Autodesk Inventor part; units mm, degrees
ref_plane "YZ Plane" through (0, 0, 0) normal (1, 0, 0) x (0, 1, 0)
ref_plane "XZ Plane" through (0, 0, 0) normal (0, 1, 0) x (-1, 0, 0)
ref_plane "XY Plane" through (0, 0, 0) normal (0, 0, 1) x (1, 0, 0)
sketch "Sketch1" plane through (0, 0, 0) normal (0, 0, 1) x (1, 0, 0)
  line L0 (0, 0) -> (-5, 0)
  line L1 (-5, 0) -> (-5, -5)
  line L2 (-5, -5) -> (0, -5)
  line L3 (0, -5) -> (0, 0)
  line L4 (-40, 0) -> (-35, 0)
  line L5 (-35, 0) -> (-35, -5)
  line L6 (-35, -5) -> (-40, -5)
  line L7 (-40, -5) -> (-40, 0)
  line L8 (0, -15.1) -> (-5, -15.1)
  line L9 (-5, -15.1) -> (-5, -10.1)
  line L10 (-5, -10.1) -> (0, -10.1)
  line L11 (0, -10.1) -> (0, -15.1)
  line L12 (-40, -15.1) -> (-35, -15.1)
  line L13 (-35, -15.1) -> (-35, -10.1)
  line L14 (-35, -10.1) -> (-40, -10.1)
  line L15 (-40, -10.1) -> (-40, -15.1)
  line L16 (0, 0) -> (-5, 0)
  line L17 (-35, 0) -> (-40, 0)
  line L18 (0, -15.1) -> (0, -10.1)
  line L19 (0, -5) -> (0, 0)
  line L20 (-40, -15.1) -> (-35, -15.1)
  line L21 (-5, -15.1) -> (0, -15.1)
  line L22 (-40, 0) -> (-40, -5)
  line L23 (-40, -10.1) -> (-40, -15.1)
  dimension "d0" = 40
  dimension "d1" = 15.1
  dimension "d2" = 5
  dimension "d3" = 5
  dimension "d4" = 5
  dimension "d5" = 5
  dimension "d6" = 5
  dimension "d7" = 5
  dimension "d8" = 5
  dimension "d9" = 5
extrude "Mounting arms" add sketch "Sketch1" along normal blind 15
sketch "Sketch2" plane through (0, 0, 0) normal (0, 0, -1) x (-1, 0, 0)
  line L0 (-19.9999, -1.0001) -> (59.9998, -1.0001)
  line L1 (59.9998, -1.0001) -> (59.9998, -14.0997)
  line L2 (59.9998, -14.0997) -> (-19.9999, -14.0997)
  line L3 (-19.9999, -14.0997) -> (-19.9999, -1.0001)
  point P0 (0, 0)
extrude "Plate" add sketch "Sketch2" along normal blind 2.5
sketch "Sketch3" plane through (19.9999, -14.0997, 0) normal (1, 0, 0) x (0, 0, -1)
  circle A0 centre (6, 6.5498) radius 5
  point P0 (0, 14.0997)
  dimension "d14" = 10
sketch "Sketch5" plane through (-59.9998, -14.0997, 0) normal (-1, 0, 0) x (0, 0, 1)
  circle A0 centre (-6, 6.5498) radius 5
  point P0 (0, 14.0997)
  dimension "d15" = 10
extrude "retainer1" add sketch "Sketch5" against normal blind 4
extrude "retainer2" add sketch "Sketch3" against normal blind 4
sketch "Sketch6" plane through (-59.9998, -14.0997, 0) normal (-1, 0, 0) x (0, 0, 1)
  line L0 (0, 13.0996) -> (0, 0)
  circle A0 centre (-5.9997, 6.4943) radius 3.5
  point P0 (0, 14.0997)
  dimension "d21" = 7
extrude "cyldiner shaft holes" cut sketch "Sketch6" against normal blind 80
chamfer "Chamfer1" distance 1 angle 45 2 edges at (-37.5, 0, 0) (-2.5, 0, 0)
sketch "Sketch7" plane through (0, 0, 15) normal (0, 0, 1) x (1, 0, 0)
  line L0 (-40, -1.0001) -> (-40, -5)
  line L1 (0, -14.0997) -> (0, -10.1)
  line L2 (-35, -14.0997) -> (-35, -10.1)
  line L3 (-40, -12.6005) -> (-35, -12.6005)
  line L4 (-35, -12.6005) -> (-35, -10.1)
  line L5 (-35, -10.1) -> (-40, -10.1)
  line L6 (-40, -10.1) -> (-40, -12.6005)
  line L7 (-5, -10.1) -> (-5, -15.1)
  line L8 (0, -12.6005) -> (-5, -12.6005)
  line L9 (-5, -12.6005) -> (-5, -10.1)
  line L10 (-5, -10.1) -> (0, -10.1)
  line L11 (0, -10.1) -> (0, -12.6005)
  line L12 (-5, -5) -> (0, -5)
  line L13 (0, -2.5001) -> (-5, -2.5001)
  line L14 (-5, -2.5001) -> (-5, -5)
  line L15 (-5, -5) -> (0, -5)
  line L16 (0, -5) -> (0, -2.5001)
  line L17 (-40, -2.5001) -> (-35, -2.5001)
  line L18 (-35, -2.5001) -> (-35, -5)
  line L19 (-35, -5) -> (-40, -5)
  line L20 (-40, -5) -> (-40, -2.5001)
  line L21 (-40, -2.5001) -> (-35, -2.5001)
  line L22 (-5, -2.5001) -> (0, -2.5001)
  line L23 (-40, -12.6005) -> (-40, -10.1)
  line L24 (-40, -5) -> (-40, -2.5001)
  line L25 (0, -12.6005) -> (-5, -12.6005)
  line L26 (-35, -12.6005) -> (-40, -12.6005)
  line L27 (0, -2.5001) -> (0, -5)
  line L28 (0, -10.1) -> (0, -12.6005)
  point P0 (0, 0)
extrude "Extrusion6" add sketch "Sketch7" along normal blind 5
fillet "Fillet1" radius 1 24 edges at (-35, -2.5001, 17.5) (-40, -2.5001, 17.5) (-37.5, -2.5001, 20) (-5, -2.5001, 17.5) (0, -2.5001, 17.5) (-2.5, -2.5001, 20) (0, -12.6005, 17.5) (-2.5, -12.6005, 20) (-5, -12.6005, 17.5) (-35, -12.6005, 17.5) (-37.5, -12.6005, 20) (-40, -12.6005, 17.5) (0, 0, 8) (-5, 0, 8) (-2.5, 0, 15) (-35, 0, 8) (-37.5, 0, 15) (-40, 0, 8) (0, -15.1, 7.5) (-2.5, -15.1, 15) (-5, -15.1, 7.5) (-35, -15.1, 7.5) (-37.5, -15.1, 15) (-40, -15.1, 7.5)
chamfer "Chamfer2" distance 1 angle 45 10 edges at (-37.5, -15.1, 0) (-35.2929, -14.8071, 0) (-35, -14.0999, 0) (-39.7071, -14.8071, 0) (-40, -14.0999, 0) (-2.5, -15.1, 0) (-0.2929, -14.8071, 0) (0, -14.0999, 0) (-4.7071, -14.8071, 0) (-5, -14.0999, 0)
sketch "Sketch8" plane through (-4, -2.5001, 15) normal (0, 1, 0) x (1, 0, 0)
  circle A0 centre (1.5, -2) radius 1
  circle A1 centre (-33.5, -2) radius 1
  point P0 (4, 15)
  dimension "d33" = 2
  dimension "d34" = 2
extrude "Extrusion7" cut sketch "Sketch8" against normal blind 10.2
properties part number "sccop_mount"
Read the model definition and answer for the solid it produces. Units are mm, in the model's axes. A direction names the side the tool comes from. Round coordinates to 2 decimals unless told otherwise and drop trailing zeros. Write each loop counter-clockwise with the first axis right and the second up, starting at its lowest first coordinate (ties: lowest second). Pieces come first, ordered by that corner, then holes. Notation, with made-up numbers: (9.5, -17) -> (59.5, -17) arc R19 ccw to (59.5, -13) -> close; hole circle Ø10 at (-12, 44). An arc over 180 degrees is marked (long way). Answer in a Markdown table with one row per item. Add a question column.
1) Given P1, Ø2, axis at x = 9, z = -2, coming from the -Y side; P2, Ø6, axis at y = -13, z = 8.5, coming from the -X side; P3, Ø2, axis at y = -3.5, z = 10.5, coming from the +X side; P4, Ø2.5, axis at x = -1.5, z = 8.5, coming from the +Y side, each flat-ended and moving along its own axis, determine where each tip first touches the part or whether it passes through.
2) Determine the mould class of faces 1 (the face through (20, -7, -2)), 2 (the face through (-37.04, -11.33, 17.89)), 3 (the face through (-37.04, -3.73, 17.89)), 4 (the face through (-3, -4, 20)) for opening direction Z: pulls with the +Z half, pulls with the -Z half, needs draft (parallel to the pull), parting line crosses it, or undercut.
3) Find section B-B, the plane x = -2.5. State how many separate pieces and enclosed holes the cut face has, and give its area (3 significant figures).
4) Find section A-A, the plane z = 6.5. Determine the outline of the cut face in (x, y), and give its area (3 significant figures).
5) Find section D-D, the plane x = -27. Determine the outline of the cut face in (y, z).
6) Consider line 1 (X direction, y = -3.6, z = 17); line 2 (X direction, y = -14.25, z = 14.5); line 3 (X direction, y = -12, z = 17). Determine where each line is inside the solid, lowest interval first.
7) Find section C-C, the plane z = -6. Determine the outline of the cut face in (x, y).
8) Which of the six approach directions +Z, -Z, +X, -X, +Y, -Y give full straight-line access (tool end or side, diameter ignored) to faces 5 (the face through (-38.19, -2.5, 16.08)), 6 (the face through (-5, -12, 8)), 7 (the face through (-40, -3, 8))?
Findings below:
| question | item | result |
|---|---|---|
| 1 | P1 | y = -14.1 |
| 1 | P2 | x = -40 |
| 1 | P3 | x = 0 |
| 1 | P4 | y = 0 |
| 2 | face 1 | needs draft |
| 2 | face 2 | undercut |
| 2 | face 3 | undercut |
| 2 | face 4 | pulls with the +Z half |
| 3 | separate pieces | 3 |
| 3 | enclosed holes | 0 |
| 3 | area | 196 mm² |
| 4 | outline | (-40, -14.1) arc R1 ccw to (-39, -15.1) -> (-36, -15.1) arc R1 ccw to (-35, -14.1) -> (-35, -10.1) -> (-40, -10.1) -> close; (-40, -5) -> (-35, -5) -> (-35, -1) arc R1 ccw to (-36, 0) -> (-39, 0) arc R1 ccw to (-40, -1) -> close; (-5, -14.1) arc R1 ccw to (-4, -15.1) -> (-1, -15.1) arc R1 ccw to (0, -14.1) -> (0, -10.1) -> (-5, -10.1) -> close; (-5, -5) -> (0, -5) -> (0, -1) arc R1 ccw to (-1, 0) -> (-4, 0) arc R1 ccw to (-5, -1) -> close |
| 4 | area | 98.3 mm² |
| 5 | outline | (-14.1, -2.5) -> (-7.65, -2.5) arc R3.5 cw to (-7.56, -2.5) -> (-1, -2.5) -> (-1, 0) -> (-14.1, 0) -> close |
| 6 | line 1 | -40 to -38.5, -36.5 to -35, -5 to -3.5, -1.5 to 0 |
| 6 | line 2 | -39.99 to -35.01, -4.99 to -0.01 |
| 6 | line 3 | -39.92 to -38.5, -36.5 to -35.08, -4.92 to -3.5, -1.5 to -0.08 |
| 7 | outline | (-60, -12.55) -> (-56, -12.55) -> (-56, -11.11) -> (-60, -11.11) -> close; (-60, -4.11) -> (-56, -4.11) -> (-56, -2.55) -> (-60, -2.55) -> close; (16, -12.55) -> (20, -12.55) -> (20, -11.11) -> (16, -11.11) -> close; (16, -4.11) -> (20, -4.11) -> (20, -2.55) -> (16, -2.55) -> close |
| 8 | face 5 | +Z, +X, -X, +Y |
| 8 | face 6 | +Z, +Y, -Y |
| 8 | face 7 | +Z, -X, +Y, -Y |
